```python
from build123d import *

# Parameters (mm, degrees)
SKETCH1_W           = 25
SKETCH1_H           = 47.5
SKETCH1_R           = 6.675
BOSS_EXTRUDE1_DEPTH = 6.35
CUT_EXTRUDE1_REACH  = 8.35
SKETCH2_R           = 1.5875


with BuildPart() as part:
    # Sketch1 → Boss-Extrude1 (new body)
    with BuildSketch(Plane(origin=(0, 0, 0), x_dir=(1, 0, 0), z_dir=(0, 1, 0))):
        with Locations((12.5, 23.75)):
            Rectangle(SKETCH1_W, SKETCH1_H)
        with Locations((12.5, 12.5)):
            Circle(SKETCH1_R, mode=Mode.SUBTRACT)
    extrude(amount=BOSS_EXTRUDE1_DEPTH)

    # Sketch2 → Cut-Extrude1 (cut, up to next)
    with BuildSketch(Plane(origin=(0, 6.35, 0), x_dir=(1, 0, 0), z_dir=(0, 1, 0)), mode=Mode.PRIVATE) as cut_extrude1_sk1:
        with Locations((20, 42.5)):
            Circle(SKETCH2_R)
    cut_extrude1_tool1 = extrude(cut_extrude1_sk1.sketch, amount=-CUT_EXTRUDE1_REACH, mode=Mode.PRIVATE) & part.part
    add(cut_extrude1_tool1.solids().sort_by_distance((20, 6.35, -42.5))[0], mode=Mode.SUBTRACT)
    # Sketch2 → Cut-Extrude1 (cut, up to next)
    with BuildSketch(Plane(origin=(0, 6.35, 0), x_dir=(1, 0, 0), z_dir=(0, 1, 0)), mode=Mode.PRIVATE) as cut_extrude1_sk2:
        with Locations((5, 42.5)):
            Circle(SKETCH2_R)
    cut_extrude1_tool2 = extrude(cut_extrude1_sk2.sketch, amount=-CUT_EXTRUDE1_REACH, mode=Mode.PRIVATE) & part.part
    add(cut_extrude1_tool2.solids().sort_by_distance((5, 6.35, -42.5))[0], mode=Mode.SUBTRACT)


solid = part.part
```
Input: part model. Units: mm. Frame: model coordinates. Round coordinates to 2 decimals unless told otherwise and drop trailing zeros. Loops run counter-clockwise (first coordinate to the right, second up) from the corner with the lowest first, then second, coordinate; pieces in that order, holes last. Notation, with made-up numbers: (-36.5, 57.5) -> (2.5, 57.5) arc R18 ccw to (2.5, 75.5) -> close; hole circle Ø10 at (60.5, 16.25). An arc over 180 degrees is marked (long way). Use one line per item in the form item = value. Start each with the question number.
Item 1: Mould query, pull axis X, two halves, no side actions, for faces 1 (the face through (20.85, 3.22, -43.84)), 2 (the face through (0, 3, -23)), 3 (the face through (25, 3, -23)). Classes: pulls with the +X half, pulls with the -X half, needs draft (parallel to the pull), parting line crosses it, or undercut.
Item 2: Material intervals for L1, parallel to X at y = 3.5, z = -42.5; L2, parallel to Z at x = 12.5, y = 4.5 (3 decimals); L3, parallel to Z at x = 20, y = 2.75, sorted ascending. Write a range as from..to.
Item 3: Section query A-A on z = -42.5. Return the cut outline in (x, y).
Item 4: Section query B-B on y = 1.5. Count the separate pieces of the cut face and the enclosed holes in it, then the cut area to 3 significant figures.
Item 5: Section query C-C on x = 5. Return the cut outline in (y, z), then the cut area to 3 significant figures.
Item 6: Section query D-D on z = -12.5. Return the cut outline in (x, y) (3 decimals).
Ans:
q1.face_1 = undercut
q1.face_2 = pulls with the -X half
q1.face_3 = pulls with the +X half
q2.L1 = 0..3.41, 6.59..18.41, 21.59..25
q2.L2 = -47.5..-19.175, -5.825..0
q2.L3 = -47.5..-44.09, -40.91..0
q3.outline = (0, 0) -> (3.41, 0) -> (3.41, 6.35) -> (0, 6.35) -> close; (6.59, 0) -> (18.41, 0) -> (18.41, 6.35) -> (6.59, 6.35) -> close; (21.59, 0) -> (25, 0) -> (25, 6.35) -> (21.59, 6.35) -> close
q4.separate_pieces = 1
q4.enclosed_holes = 3
q4.area = 1,030 mm^2
q5.outline = (0, -47.5) -> (6.35, -47.5) -> (6.35, -44.09) -> (0, -44.09) -> close; (0, -40.91) -> (6.35, -40.91) -> (6.35, 0) -> (0, 0) -> close
q5.area = 281 mm^2
q6.outline = (0, 0) -> (5.825, 0) -> (5.825, 6.35) -> (0, 6.35) -> close; (19.175, 0) -> (25, 0) -> (25, 6.35) -> (19.175, 6.35) -> close
